Could you check a few things on this model? Use its own coordinates, in mm. A direction names the side the tool comes from. Give positions to 0.01 mm unless a question says otherwise; leave off trailing zeros. Loops run counter-clockwise (first coordinate to the right, second up) from the corner with the lowest first, then second, coordinate; pieces in that order, holes last. Notation, with made-up numbers: (1, 19) -> (23, 19) arc R22 ccw to (23, 55) -> close; hole circle Ø5 at (83.5, -37.5). An arc over 180 degrees is marked (long way). Write item = value, one per line. Start each with the question number.
1) I'm going to push flat-ended pins straight in: pin 1 Ø4 at (x, y) = (-47, 68.5) entering from +Z; pin 2 Ø24 at (x, y) = (0, 0) entering from +Z; pin 3 Ø4 at (y, z) = (110.5, 82.5) entering from -X; pin 4 Ø3 at (x, y) = (-121.5, 109.5) entering from +Z. Where does each tip first touch, or does it pass through?
2) On a 3-axis mill with a long thin cutter (end or side, diameter ignored), from which of +Z, -Z, +X, -X, +Y, -Y can I reach the whole of each face in a straight line? I mean faces 3 (the face through (2.067, 149.55, 123.045)), 4 (the face through (-94, 218, 430)), 5 (the face through (1, 21, 10)). Say none if no direction works.
3) I want a section at B-B (x = 26). List the corners of the cut face in (y, z) for me.
4) I want a section at C-C (x = -60). List the corners of the cut face in (y, z) for me, and give its area (3 significant figures).
5) I want a section at A-A (z = 70). List the corners of the cut face in (x, y) for me, and give its area (3 significant figures).
6) I need wall thicknesses on probe 1 along Z at (x, y) = (59, -5); probe 2 along X at (y, z) = (114, 169); probe 3 along Z at (x, y) = (-14, 116). Which ranges of each line are inside material? Lowest first, please. Write a range as from..to.
7) I want a section at D-D (y = 121). Count the separate pieces of the cut face and the enclosed holes in it, and give its area (3 significant figures).
8) If we mould it in two halves opening along Z, with no side actions, what happens to faces 1 (the face through (-14.985, 0.66, 437.395)), 2 (the face through (109, 153, 120))? For each: +Z half, -Z half, draft (parallel to the pull), parting line (faces both ways), or undercut.
from build123d import *

# Parameters (mm, degrees)
SKETCH1_R                = 15
BOSS_EXTRUDE1_DEPTH      = 10
SKETCH2_W                = 200
SKETCH2_H                = 150
BOSS_EXTRUDE2_DEPTH      = 420
SKETCH3_R                = 47
CUT_EXTRUDE1_DEPTH       = 150
CHAMFER2_SIZE            = 15
BOSS_EXTRUDE3_START      = 10
BOSS_EXTRUDE3_DEPTH      = 420
BOSS_EXTRUDE4_DEPTH      = 5
BOSS_EXTRUDE4_DEPTH_BACK = 5
BOSS_EXTRUDE4_START      = 115
SKETCH5_W                = 39.105801637
SKETCH5_H                = 223.5
BOSS_EXTRUDE5_DEPTH      = 5
BOSS_EXTRUDE5_DEPTH_BACK = 5
BOSS_EXTRUDE5_START      = 325
SKETCH5_3_W              = 39.105801637
SKETCH5_3_H              = 223.5
BOSS_EXTRUDE6_DEPTH      = 10
BOSS_EXTRUDE6_DEPTH_BACK = 10
BOSS_EXTRUDE6_START      = 115
SKETCH5_4_W              = 6
SKETCH5_4_H              = 223.5
BOSS_EXTRUDE7_DEPTH      = 10
BOSS_EXTRUDE7_DEPTH_BACK = 10
BOSS_EXTRUDE7_START      = 325
SKETCH5_5_W              = 6
SKETCH5_5_H              = 223.5
SKETCH10_R               = 15
BOSS_EXTRUDE8_DEPTH      = 10
SKETCH10_3_R             = 20
SKETCH10_3_R_2           = 15
BOSS_EXTRUDE9_DEPTH      = 15


with BuildPart() as part:
    # Sketch1 → Boss-Extrude1 (new body)
    with BuildSketch(Plane.XY):
        with BuildLine():
            Line((-100, 73.5), (-100, 223.5))
            Line((-100, 223.5), (100, 223.5))
            Line((100, 223.5), (100, 73.5))
            ThreePointArc((100, 73.5), (124.013298207, 4.790810776), (105.372324855, -65.566173861))
            ThreePointArc((105.372324855, -65.566173861), (98.104066029, -72.483184453), (88.39127748, -75))
            Line((88.39127748, -75), (-88.39127748, -75))
            ThreePointArc((-88.39127748, -75), (-98.104066029, -72.483184453), (-105.372324855, -65.566173861))
            ThreePointArc((-105.372324855, -65.566173861), (-124.013298207, 4.790810776), (-100, 73.5))
        make_face()
        Circle(SKETCH1_R, mode=Mode.SUBTRACT)
    extrude(amount=BOSS_EXTRUDE1_DEPTH)



with BuildPart() as body_2:
    # Sketch2 → Boss-Extrude2 (new body)
    with BuildSketch(Plane.XY.offset(10)):
        with Locations((0, 148.5)):
            Rectangle(SKETCH2_W, SKETCH2_H)
    extrude(amount=BOSS_EXTRUDE2_DEPTH)

    # Sketch3 → Cut-Extrude1 (cut)
    with BuildSketch(Plane(origin=(0, 223.5, 0), x_dir=(1, 0, 0), z_dir=(0, 1, 0))):
        with Locations(Location((0, -370, 0), (0, 0, 270))):
            Circle(SKETCH3_R)
        with Locations(Location((0, -270, 0), (0, 0, 270))):
            Circle(SKETCH3_R)
        with Locations(Location((0, -170, 0), (0, 0, 270))):
            Circle(SKETCH3_R)
        with Locations(Location((0, -70, 0), (0, 0, 270))):
            Circle(SKETCH3_R)
    extrude(amount=-CUT_EXTRUDE1_DEPTH, mode=Mode.SUBTRACT)

    # Chamfer2
    chamfer2_edges = [body_2.edges().sort_by_distance(p)[0] for p in [
        (-100, 223.5, 220),
        (100, 223.5, 220),
    ]]
    chamfer(chamfer2_edges, length=CHAMFER2_SIZE)


with BuildPart() as part_1:
    add(part.part)

    add(body_2.part)  # Boss-Extrude3 merges body 2
    # Sketch4 → Boss-Extrude3 (add)
    with BuildSketch(Plane.XY.offset(BOSS_EXTRUDE3_START)):
        with BuildLine():
            Line((88.39127748, -75), (-88.39127748, -75))
            ThreePointArc((-88.39127748, -75), (-98.104066029, -72.483184453), (-105.372324855, -65.566173861))
            ThreePointArc((-105.372324855, -65.566173861), (-124.013298207, 4.790810776), (-100, 73.5))
            Line((-100, 73.5), (-55, 73.5))
            ThreePointArc((-55, 73.5), (-62.071067812, 70.571067812), (-65, 63.5))
            Line((-65, 63.5), (-65, 0))
            ThreePointArc((-65, 0), (0, -65), (65, 0))
            Line((65, 0), (65, 63.5))
            ThreePointArc((65, 63.5), (62.071067812, 70.571067812), (55, 73.5))
            Line((55, 73.5), (100, 73.5))
            ThreePointArc((100, 73.5), (124.013298207, 4.790810776), (105.372324855, -65.566173861))
            ThreePointArc((105.372324855, -65.566173861), (98.104066029, -72.483184453), (88.39127748, -75))
        make_face()
    extrude(amount=BOSS_EXTRUDE3_DEPTH)

    # Sketch5 → Boss-Extrude4 (add, two sides: drawn at the far end of the back side and taken through both)
    with BuildSketch(Plane.XY.offset(BOSS_EXTRUDE4_START - BOSS_EXTRUDE4_DEPTH_BACK)):
        with Locations((-104.552900819, 111.75)):
            Rectangle(SKETCH5_W, SKETCH5_H)
        with Locations((104.552900819, 111.75)):
            Rectangle(SKETCH5_W, SKETCH5_H)
    extrude(amount=BOSS_EXTRUDE4_DEPTH + BOSS_EXTRUDE4_DEPTH_BACK)

    # Sketch5_3 → Boss-Extrude5 (add, two sides: drawn at the far end of the back side and taken through both)
    with BuildSketch(Plane.XY.offset(BOSS_EXTRUDE5_START - BOSS_EXTRUDE5_DEPTH_BACK)):
        with Locations((-104.552900819, 111.75)):
            Rectangle(SKETCH5_3_W, SKETCH5_3_H)
        with Locations((104.552900819, 111.75)):
            Rectangle(SKETCH5_3_W, SKETCH5_3_H)
    extrude(amount=BOSS_EXTRUDE5_DEPTH + BOSS_EXTRUDE5_DEPTH_BACK)

    # Sketch5_4 → Boss-Extrude6 (add, two sides: drawn at the far end of the back side and taken through both)
    with BuildSketch(Plane.XY.offset(BOSS_EXTRUDE6_START - BOSS_EXTRUDE6_DEPTH_BACK)):
        with Locations((121.105801637, 111.75)):
            Rectangle(SKETCH5_4_W, SKETCH5_4_H)
        with Locations((-121.105801637, 111.75)):
            Rectangle(SKETCH5_4_W, SKETCH5_4_H)
    extrude(amount=BOSS_EXTRUDE6_DEPTH + BOSS_EXTRUDE6_DEPTH_BACK)

    # Sketch5_5 → Boss-Extrude7 (add, two sides: drawn at the far end of the back side and taken through both)
    with BuildSketch(Plane.XY.offset(BOSS_EXTRUDE7_START - BOSS_EXTRUDE7_DEPTH_BACK)):
        with Locations((-121.105801637, 111.75)):
            Rectangle(SKETCH5_5_W, SKETCH5_5_H)
        with Locations((121.105801637, 111.75)):
            Rectangle(SKETCH5_5_W, SKETCH5_5_H)
    extrude(amount=BOSS_EXTRUDE7_DEPTH + BOSS_EXTRUDE7_DEPTH_BACK)

    # Sketch10 → Boss-Extrude8 (add)
    with BuildSketch(Plane.XY.offset(430)):
        with BuildLine():
            Line((100, 223.5), (-100, 223.5))
            Line((-100, 223.5), (-100, 73.5))
            ThreePointArc((-100, 73.5), (-124.013298207, 4.790810776), (-105.372324855, -65.566173861))
            ThreePointArc((-105.372324855, -65.566173861), (-98.104066029, -72.483184453), (-88.39127748, -75))
            Line((-88.39127748, -75), (88.39127748, -75))
            ThreePointArc((88.39127748, -75), (98.104066029, -72.483184453), (105.372324855, -65.566173861))
            ThreePointArc((105.372324855, -65.566173861), (124.013298207, 4.790810776), (100, 73.5))
            Line((100, 73.5), (100, 223.5))
        make_face()
        Circle(SKETCH10_R, mode=Mode.SUBTRACT)
    extrude(amount=BOSS_EXTRUDE8_DEPTH)

    # Sketch10_3 → Boss-Extrude9 (add)
    with BuildSketch(Plane.XY.offset(430)):
        Circle(SKETCH10_3_R)
        Circle(SKETCH10_3_R_2, mode=Mode.SUBTRACT)
    extrude(amount=BOSS_EXTRUDE9_DEPTH)


solid = part_1.part
Answer list:
q1.pin_1 = 440
q1.pin_2 = through
q1.pin_3 = -100
q1.pin_4 = 335
q2.face_3 = +Y
q2.face_4 = -X, +Y
q2.face_5 = none
q3.outline = (-75, 0) -> (223.5, 0) -> (223.5, 30.85) -> (73.5, 30.85) -> (73.5, 10) -> (-59.57, 10) -> (-59.57, 430) -> (73.5, 430) -> (73.5, 409.15) -> (223.5, 409.15) -> (223.5, 440) -> (-75, 440) -> close; (73.5, 109.15) -> (223.5, 109.15) -> (223.5, 130.85) -> (73.5, 130.85) -> close; (73.5, 209.15) -> (223.5, 209.15) -> (223.5, 230.85) -> (73.5, 230.85) -> close; (73.5, 309.15) -> (223.5, 309.15) -> (223.5, 330.85) -> (73.5, 330.85) -> close
q4.outline = (-75, 0) -> (223.5, 0) -> (223.5, 440) -> (-75, 440) -> close; hole (-25, 10) -> (72.16, 10) -> (72.16, 430) -> (-25, 430) -> close
q4.area = 90,500 mm^2
q5.outline = (-105.37, -65.57) arc R20 ccw to (-88.39, -75) -> (88.39, -75) arc R20 ccw to (105.37, -65.57) arc R124.11 ccw to (100, 73.5) -> (100, 208.5) -> (85, 223.5) -> (47, 223.5) -> (47, 73.5) -> (55, 73.5) arc R10 cw to (65, 63.5) -> (65, 0) arc R65 cw to (-65, 0) -> (-65, 63.5) arc R10 cw to (-55, 73.5) -> (-47, 73.5) -> (-47, 223.5) -> (-85, 223.5) -> (-100, 208.5) -> (-100, 73.5) arc R124.11 ccw to start
q5.area = 34,000 mm^2
q6.probe_1 = 0..10, 430..440
q6.probe_2 = -100..-46.99, 46.99..100
q6.probe_3 = 0..25.13, 114.87..125.13, 214.87..225.13, 314.87..325.13, 414.87..440
q7.separate_pieces = 1
q7.enclosed_holes = 4
q7.area = 61,400 mm^2
q8.face_1 = draft
q8.face_2 = undercut
